Can you work these out from the model? Positions are in its coordinate system, mm. A direction names the side the tool comes from. Give positions to 0.01 mm unless a question says otherwise; leave off trailing zeros. Write each loop counter-clockwise with the first axis right and the second up, starting at its lowest first coordinate (ties: lowest second). Pieces come first, ordered by that corner, then holes.
```python
from build123d import *

# Parameters (mm, degrees)
SKETCH1_W                               = 60
SKETCH1_H                               = 38
BASE_DEPTH                              = 13
ADDALITTLEBEAUTY_R                      = 8
SKETCH1_3_R                             = 9
RODHOLDER_DEPTH                         = 20
M5X0_8_TAPPED_HOLE_FOR_FIXING_ROD_D     = 4.2
M5X0_8_TAPPED_HOLE_FOR_FIXING_ROD_DEPTH = 10.4
M5X0_8_TAPPED_HOLE_FOR_FIXING_ROD_TIP   = 1.2618073
CHAMFER1_SIZE                           = 4
F_10_2_10_2_ROD_HOLE_D                  = 10.2
M3X0_5_TAPPED_HOLE1_D                   = 2.5
M3X0_5_TAPPED_HOLE1_CSINK_D             = 3.05
M3X0_5_TAPPED_HOLE1_CSINK_ANGLE         = 90
SKETCH9_W                               = 27
SKETCH9_H                               = 27
CUT_EXTRUDE1_DEPTH                      = 9
FILLET1_R                               = 2


with BuildPart() as part:
    # Sketch1 → Base (new body)
    with BuildSketch(Plane(origin=(0, 0, 0), x_dir=(1, 0, 0), z_dir=(0, 1, 0))):
        with Locations((-19, 0)):
            Rectangle(SKETCH1_W, SKETCH1_H)
    extrude(amount=BASE_DEPTH)

    # AddALittleBeauty
    addalittlebeauty_edges = [part.edges().sort_by_distance(p)[0] for p in [
        (11, 6.5, -19),
        (11, 6.5, 19),
        (-49, 6.5, 19),
        (-49, 6.5, -19),
    ]]
    fillet(addalittlebeauty_edges, radius=ADDALITTLEBEAUTY_R)

    # Sketch1<3> → RodHolder (add)
    with BuildSketch(Plane(origin=(0, 0, 0), x_dir=(1, 0, 0), z_dir=(0, 1, 0))):
        with Locations(Location((0, 0, 0), (0, 0, 270))):
            Circle(SKETCH1_3_R)
    extrude(amount=RODHOLDER_DEPTH)

    # M5x0.8 Tapped Hole for fixing rod
    with Locations(Plane(origin=(11, 0, 0), x_dir=(0, 0, -1), z_dir=(1, 0, 0))):
        with Locations((0, 6)):
            Hole(M5X0_8_TAPPED_HOLE_FOR_FIXING_ROD_D / 2, depth=M5X0_8_TAPPED_HOLE_FOR_FIXING_ROD_DEPTH)
            with Locations((0, 0, -(M5X0_8_TAPPED_HOLE_FOR_FIXING_ROD_DEPTH + M5X0_8_TAPPED_HOLE_FOR_FIXING_ROD_TIP / 2))):  # 118° drill point
                Cone(0, M5X0_8_TAPPED_HOLE_FOR_FIXING_ROD_D / 2, M5X0_8_TAPPED_HOLE_FOR_FIXING_ROD_TIP, mode=Mode.SUBTRACT)

    # Chamfer1
    # the kernel refuses this chamfer: 4 mm, written as the material it adds along each edge
    with BuildSketch(Plane(origin=(0, 13, 0), x_dir=(0, 0, 1), z_dir=(1, 0, 0))) as chamfer1_piece_1_section:
        Polygon((9 + CHAMFER1_SIZE, 0), (9, -CHAMFER1_SIZE), (9, 0), align=None)
    chamfer1_piece_1 = revolve(axis=Axis((0, 13, 0), (0, -1, 0)), mode=Mode.PRIVATE)
    chamfer1_piece_1 = split(chamfer1_piece_1, bisect_by=Plane(origin=(11, 14.941949716, -10.941949716), z_dir=(-1, 0, 0)), keep=Keep.TOP, mode=Mode.PRIVATE)
    add(chamfer1_piece_1)

    # Ø10.2 (10.2) Rod Hole (through all)
    with Locations(Plane(origin=(0, 20, 0), x_dir=(1, 0, 0), z_dir=(0, 1, 0))):
        with Locations((0, 0)):
            Hole(F_10_2_10_2_ROD_HOLE_D / 2)

    # M3x0.5 Tapped Hole1 (through all)
    with Locations(Plane(origin=(0, 0, 0), x_dir=(-1, 0, 0), z_dir=(0, -1, 0))):
        with Locations((-6, 14), (-6, -14), (44, -14), (44, 14), (10, 14), (10, -14)):
            CounterSinkHole(M3X0_5_TAPPED_HOLE1_D / 2, M3X0_5_TAPPED_HOLE1_CSINK_D / 2, counter_sink_angle=M3X0_5_TAPPED_HOLE1_CSINK_ANGLE)

    # Sketch9 → Cut-Extrude1 (cut)
    with BuildSketch(Plane.XZ):
        with Locations((-27, 0)):
            Rectangle(SKETCH9_W, SKETCH9_H)
    extrude(amount=-CUT_EXTRUDE1_DEPTH, mode=Mode.SUBTRACT)

    # Fillet1
    fillet1_edges = [part.edges().sort_by_distance(p)[0] for p in [
        (-40.5, 9, 0),
        (-40.5, 4.5, -13.5),
        (-27, 9, 13.5),
        (-40.5, 4.5, 13.5),
        (-13.5, 9, 0),
        (-13.5, 4.5, 13.5),
        (-27, 9, -13.5),
        (-13.5, 4.5, -13.5),
    ]]
    fillet(fillet1_edges, radius=FILLET1_R)


solid = part.part
```
1) For pin 1 Ø4 at (x, z) = (6, -14) entering from +Y; pin 2 Ø1.5 at (y, z) = (16, 0.5) entering from -X; pin 3 Ø11.5 at (x, z) = (-28.5, 3.5) entering from -Y, each with a flat end and sliding along its axis, tell me the tip position at first contact or that it passes through.
Values follow:
pin 1: stops at y = 13
pin 2: stops at x = -10.74
pin 3: stops at y = 9
2) Suppose I cut it at C-C on y = 19. Write out the boundary of the cut face in (x, z).
Values follow:
outline: circle Ø18 at (0, 0); hole circle Ø10.2 at (0, 0)
3) If we mould it in two halves opening along X, with no side actions, what happens to faces 3 (the face through (-27, 3, 13.5)), 4 (the face through (-39.93, 8.4, 0.16)), 5 (the face through (-46.719, 6.591, 16.594)), 6 (the face through (-19, 6, 19))? For each: +X half, -X half, draft (parallel to the pull), parting line (faces both ways), or undercut.
Values follow:
face 3: undercut
face 4: undercut
face 5: -X half
face 6: draft
4) Suppose I cut it at B-B on y = 6. Write out the boundary of the cut face in (x, z).
Values follow:
outline: (-49, -11) arc R8 ccw to (-41, -19) - (3, -19) arc R8 ccw to (11, -11) - (11, -2.1) - (4.65, -2.1) arc R5.1 cw (long way) to (4.65, 2.1) - (11, 2.1) - (11, 11) arc R8 ccw to (3, 19) - (-41, 19) arc R8 ccw to (-49, 11) - close; hole circle Ø2.5 at (-44, -14); hole circle Ø2.5 at (-44, 14); hole (-40.5, -11.5) arc R2 ccw to (-38.5, -13.5) - (-15.5, -13.5) arc R2 ccw to (-13.5, -11.5) - (-13.5, 11.5) arc R2 ccw to (-15.5, 13.5) - (-38.5, 13.5) arc R2 ccw to (-40.5, 11.5) - close; hole circle Ø2.5 at (-10, -14); hole circle Ø2.5 at (-10, 14); hole circle Ø2.5 at (6, -14); hole circle Ø2.5 at (6, 14)
5) Please list where these lines run through material, in increasing order: L1, parallel to Z at x = -10, y = 8.25; L2, parallel to X at y = 7.75, z = 14; L3, parallel to X at y = 3.5, z = -11.
Values follow:
L1: z = -19 to -15.25, -12.75 to 12.75, 15.25 to 19
L2: x = -48.42 to -45.25, -42.75 to -11.25, -8.75 to 4.75, 7.25 to 10.42
L3: x = -49 to -40.5, -13.5 to 11
6) For faces 1 (the face through (-39.93, 3.55, -12.9)), 2 (the face through (-10.921, 6.727, 13.155)), which set-ups out of +Z, -Z, +X, -X, +Y, -Y let a thin tool reach every point of the face, with its end or its side?
Values follow:
face 1: -Y
face 2: +Y, -Y
7) Suppose I cut it at A-A on z = 0. Write out the boundary of the cut face in (x, y), plus the area to 3 significant figures.
Values follow:
outline: (-49, 0) - (-40.5, 0) - (-40.5, 7) arc R2 cw to (-38.5, 9) - (-15.5, 9) arc R2 cw to (-13.5, 7) - (-13.5, 0) - (-5.1, 0) - (-5.1, 20) - (-9, 20) - (-9, 17) - (-13, 13) - (-49, 13) - close; (5.1, 0) - (11, 0) - (11, 3.9) - (5.1, 3.9) - close; (5.1, 8.1) - (11, 8.1) - (11, 15) - (9, 17) - (9, 20) - (5.1, 20) - close
area: 450 mm2
8) Suppose I cut it at D-D on x = 6. State how many separate pieces and enclosed holes the cut face has, plus the area to 3 significant figures.
Values follow:
separate pieces: 3
enclosed holes: 1
area: 514 mm2
